Can you work these out from the model? Positions are in its coordinate system, mm. Coordinates: 2 decimals unless noted, no trailing zeros. Order: outer loops, then holes, each group sorted by start corner. A loop starts at its lowest first (then second) coordinate and runs counter-clockwise, first axis right, second up. Notation, with made-up numbers: (75.5, 81) - (107.5, 81) arc R30 cw to (107.5, 114) - close; hole circle Ø1 at (2, 40.5). An arc over 180 degrees is marked (long way). Return JSON: item names as keys, results as strings. Group by question number.
1) For pin 1 Ø2 at (y, z) = (7, -56.5) entering from -X; pin 2 Ø5 at (x, z) = (79.5, -10.5) entering from +Y, each with a flat end and sliding along its axis, tell me the tip position at first contact or that it passes through.
2) Imagine slicing it at D-D (z = -12). Write out the boundary of the cut face in (x, y), and give its area (3 significant figures).
3) Imagine slicing it at C-C (z = -59.5). Write out the boundary of the cut face in (x, y), and give its area (3 significant figures).
4) Imagine slicing it at B-B (x = 29.5). Write out the boundary of the cut face in (y, z).
5) If I drill on line 1 along X through (y, z) = (6.75, -59.5); line 2 along X through (y, z) = (3.25, -3.5); line 3 along Z through (x, y) = (143.5, 2.5), over which ranges is the centre line in solid material (lowest first)?
6) Imagine slicing it at A-A (z = -3.5). Write out the boundary of the cut face in (x, y).
```python
from build123d import *

# Parameters (mm, degrees)
SKIZZE3_W                       = 147
SKIZZE3_H                       = 63
AUFSATZ_LINEAR_AUSTRAGEN2_DEPTH = 2
SKIZZE4_W                       = 124
SKIZZE4_H                       = 43
SCHNITT_LINEAR_AUSTRAGEN1_DEPTH = 2
SKIZZE5_R                       = 2.752378696
AUFSATZ_LINEAR_AUSTRAGEN3_DEPTH = 9.4
SKIZZE6_R                       = 1.6
SCHNITT_LINEAR_AUSTRAGEN2_DEPTH = 11.4
SKIZZE7_R                       = 2.5
AUFSATZ_LINEAR_AUSTRAGEN4_DEPTH = 9.4
SKIZZE8_R                       = 1.6
SCHNITT_LINEAR_AUSTRAGEN3_DEPTH = 11.4
SKIZZE9_R                       = 2.5
AUFSATZ_LINEAR_AUSTRAGEN5_DEPTH = 9.4


with BuildPart() as part:
    # Skizze3 → Aufsatz-Linear austragen2 (new body)
    with BuildSketch(Plane(origin=(0, 0, 0), x_dir=(1, 0, 0), z_dir=(0, 1, 0))):
        with Locations((73.5, 31.5)):
            Rectangle(SKIZZE3_W, SKIZZE3_H)
    extrude(amount=AUFSATZ_LINEAR_AUSTRAGEN2_DEPTH)

    # Skizze4 → Schnitt-Linear austragen1 (cut)
    with BuildSketch(Plane(origin=(0, 2, 0), x_dir=(1, 0, 0), z_dir=(0, 1, 0))):
        with Locations((73.5, 30.5)):
            Rectangle(SKIZZE4_W, SKIZZE4_H)
    extrude(amount=-SCHNITT_LINEAR_AUSTRAGEN1_DEPTH, mode=Mode.SUBTRACT)

    # Skizze5 → Aufsatz-Linear austragen3 (add)
    with BuildSketch(Plane(origin=(0, 2, 0), x_dir=(1, 0, 0), z_dir=(0, 1, 0))):
        with Locations(Location((3.5, 59.5, 0), (0, 0, 270))):
            Circle(SKIZZE5_R)
    extrude(amount=AUFSATZ_LINEAR_AUSTRAGEN3_DEPTH)

    # Skizze6 → Schnitt-Linear austragen2 (cut)
    with BuildSketch(Plane(origin=(0, 11.4, 0), x_dir=(1, 0, 0), z_dir=(0, 1, 0))):
        with Locations(Location((3.5, 59.5, 0), (0, 0, 270))):
            Circle(SKIZZE6_R)
    extrude(amount=-SCHNITT_LINEAR_AUSTRAGEN2_DEPTH, mode=Mode.SUBTRACT)

    # Skizze7 → Aufsatz-Linear austragen4 (add)
    with BuildSketch(Plane(origin=(0, 2, 0), x_dir=(1, 0, 0), z_dir=(0, 1, 0))):
        with Locations(Location((143.5, 3.5, 0), (0, 0, 270))):
            Circle(SKIZZE7_R)
    extrude(amount=AUFSATZ_LINEAR_AUSTRAGEN4_DEPTH)

    # Skizze8 → Schnitt-Linear austragen3 (cut)
    with BuildSketch(Plane(origin=(0, 11.4, 0), x_dir=(1, 0, 0), z_dir=(0, 1, 0))):
        with Locations(Location((143.5, 3.5, 0), (0, 0, 270))):
            Circle(SKIZZE8_R)
    extrude(amount=-SCHNITT_LINEAR_AUSTRAGEN3_DEPTH, mode=Mode.SUBTRACT)

    # Skizze9 → Aufsatz-Linear austragen5 (add)
    with BuildSketch(Plane(origin=(0, 2, 0), x_dir=(1, 0, 0), z_dir=(0, 1, 0))):
        with Locations(Location((143.5, 59.5, 0), (0, 0, 270))):
            Circle(SKIZZE9_R)
        with Locations(Location((3.5, 3.5, 0), (0, 0, 270))):
            Circle(SKIZZE9_R)
    extrude(amount=AUFSATZ_LINEAR_AUSTRAGEN5_DEPTH)


solid = part.part
```
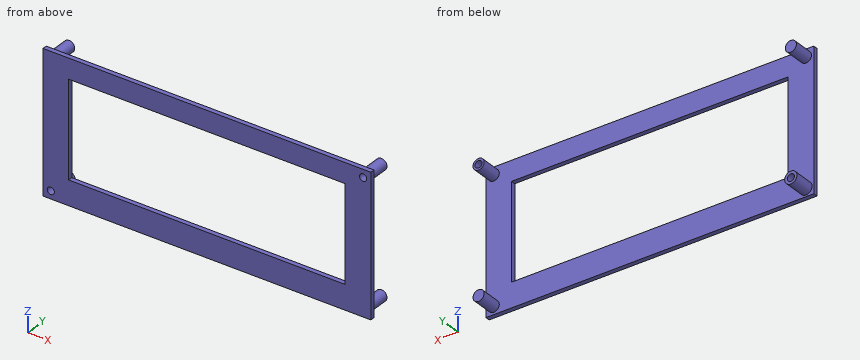
Calculated:
{
 "1": {"pin 1": "x = 1.61", "pin 2": "y = 2"},
 "2": {"outline": "(0, 0) - (11.5, 0) - (11.5, 2) - (0, 2) - close; (135.5, 0) - (147, 0) - (147, 2) - (135.5, 2) - close", "area": "46.0 mm2"},
 "3": {"outline": "(0, 0) - (1.9, 0) - (1.9, 11.4) - (0.75, 11.4) - (0.75, 2) - (0, 2) - close; (5.1, 0) - (147, 0) - (147, 2) - (146, 2) - (146, 11.4) - (141, 11.4) - (141, 2) - (6.25, 2) - (6.25, 11.4) - (5.1, 11.4) - close", "area": "356 mm2"},
 "4": {"outline": "(0, -63) - (2, -63) - (2, -52) - (0, -52) - close; (0, -9) - (2, -9) - (2, 0) - (0, 0) - close"},
 "5": {"line 1": "0.75 to 1.9, 5.1 to 6.25, 141 to 146", "line 2": "1 to 6, 141 to 141.9, 145.1 to 146", "line 3": "-62 to -57, -6 to -5.1, -1.9 to -1"},
 "6": {"outline": "(0, 0) - (141.9, 0) - (141.9, 11.4) - (141, 11.4) - (141, 2) - (6, 2) - (6, 11.4) - (1, 11.4) - (1, 2) - (0, 2) - close; (145.1, 0) - (147, 0) - (147, 2) - (146, 2) - (146, 11.4) - (145.1, 11.4) - close"}
}
